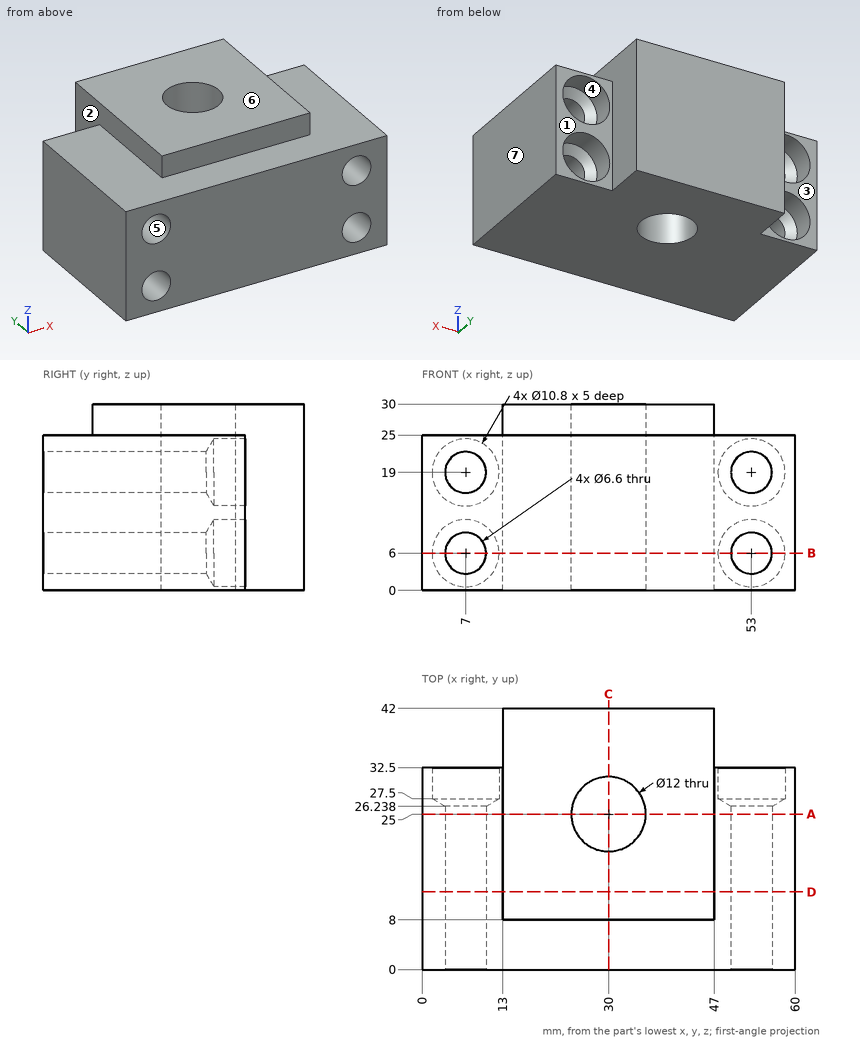
Study the drawing (mm; zero at the part's minimum x, y, z) and answer. A direction names the side the tool comes from. Coordinates: 2 decimals unless noted, no trailing zeros. Write each loop counter-clockwise with the first axis right and the second up, starting at its lowest first coordinate (ties: lowest second). Pieces come first, ordered by that corner, then holes. Notation, with made-up numbers: M 34,64 L 46,64 A5 ccw 46,70 Z; hole C 9,5.5 d2. An arc over 180 degrees is marked long. Use one line per item in the form item = value.
Item 1: The mould has two halves that part along X. Classify the marked faces 5, 6 and 7: released by +X, released by -X, zero draft, split by the parting line, or undercut.
Model answer:
face_5 = undercut
face_6 = zero draft
face_7 = released by +X
Item 2: Find section C-C, the plane x = 30. Give the vertices of the cut face in (y, z).
Model answer:
outline = M 0,0 L 19,0 L 19,30 L 8,30 L 8,25 L 0,25 Z; M 31,0 L 42,0 L 42,30 L 31,30 Z
Item 3: Find section D-D, the plane y = 12.5. Give the vertices of the cut face in (x, z).
Model answer:
outline = M 0,0 L 60,0 L 60,25 L 47,25 L 47,30 L 13,30 L 13,25 L 0,25 Z; hole C 7,6 d6.6; hole C 7,19 d6.6; hole C 53,6 d6.6; hole C 53,19 d6.6
Item 4: Find section A-A, the plane y = 25. Give the vertices of the cut face in (x, z).
Model answer:
outline = M 0,0 L 24,0 L 24,30 L 13,30 L 13,25 L 0,25 Z; M 36,0 L 60,0 L 60,25 L 47,25 L 47,30 L 36,30 Z; hole C 7,6 d6.6; hole C 7,19 d6.6; hole C 53,6 d6.6; hole C 53,19 d6.6
Item 5: For the marked faces 1, 2, 3 and 4, determine the directions among +Z, -Z, +X, -X, +Y, -Y from which every point of the face is accessible in a straight line to the end or side of a thin tool.
Model answer:
face_1 = +Z, -Z, +X, +Y
face_2 = +Z, -X, +Y
face_3 = +Z, -Z, -X, +Y
face_4 = +Y
Item 6: Find section B-B, the plane z = 6. Give the vertices of the cut face in (x, y), plus the area to 3 significant figures.
Model answer:
outline = M 0,0 L 3.7,0 L 3.7,26.24 L 1.6,27.5 L 1.6,32.5 L 0,32.5 Z; M 10.3,0 L 49.7,0 L 49.7,26.24 L 47.6,27.5 L 47.6,32.5 L 47,32.5 L 47,42 L 13,42 L 13,32.5 L 12.4,32.5 L 12.4,27.5 L 10.3,26.24 Z; M 56.3,0 L 60,0 L 60,32.5 L 58.4,32.5 L 58.4,27.5 L 56.3,26.24 Z; hole C 30,25 d12
area = 1,680 mm2
Item 7: Find the intervals of material crossed by probe 1 along Z at (x, y) = (7, 28); probe 2 along Z at (x, y) = (7, 20); probe 3 along X at (y, z) = (5, 19.25), in increasing order.
Model answer:
probe_1 = 0 to 0.6, 11.4 to 13.6, 24.4 to 25
probe_2 = 0 to 2.7, 9.3 to 15.7, 22.3 to 25
probe_3 = 0 to 3.71, 10.29 to 49.71, 56.29 to 60
Item 8: Given P1, Ø6, axis at x = 7, z = 6, coming from the -Y side; P2, Ø8.5, axis at x = 7, z = 6, coming from the +Y side; P3, Ø14.5, axis at x = 56, z = 16, coming from the +Y side; P4, Ø4, axis at x = 38.5, z = 28.5, coming from the -Y side, each flat-ended and moving along its own axis, determine where each tip first touches the part or whether it passes through.
Model answer:
P1 = through
P2 = 26.81
P3 = 32.5
P4 = 8
